Geometry check sheet. Reference: the model listing, model coordinates, mm. A direction names the side the tool comes from. Round coordinates to 2 decimals unless told otherwise and drop trailing zeros. Write each loop counter-clockwise with the first axis right and the second up, starting at its lowest first coordinate (ties: lowest second). Pieces come first, ordered by that corner, then holes. Notation, with made-up numbers: M 40,27 L 56,27 A13 cw 56,50 Z; hole C 56.5,63.5 d8. An arc over 180 degrees is marked long. Answer as CSV lines item,"result". Start each with the question number.
Autodesk Inventor part; units mm, degrees
ref_plane "YZ Plane" through (0, 0, 0) normal (1, 0, 0) x (0, 1, 0)
ref_plane "XZ Plane" through (0, 0, 0) normal (0, 1, 0) x (-1, 0, 0)
ref_plane "XY Plane" through (0, 0, 0) normal (0, 0, 1) x (1, 0, 0)
sketch "Skizze1" plane through (0, 0, 0) normal (0, 0, 1) x (1, 0, 0)
  line L0 (-7, 0) -> (7, 0)
  line L1 (0, -7) -> (0, 7)
  circle A0 centre (0, 0) radius 5
  dimension "d0" = 10
extrude "Extrusion1" add sketch "Skizze1" along normal mid plane 25
sketch "Skizze2" plane through (0, 0, -12.5) normal (0, 0, -1) x (-1, 0, 0)
  circle A0 centre (0, 0) radius 2.5
  dimension "d3" = 5
extrude "Extrusion2" add sketch "Skizze2" along normal blind 15
sketch "Skizze3" plane through (0, 0, 12.5) normal (0, 0, 1) x (1, 0, 0)
  circle A0 centre (0, 0) radius 2.5
  circle A1 centre (0, 0) radius 2.5
extrude "Extrusion3" add sketch "Skizze3" along normal blind 15
thread "Gewinde1"
sketch "Skizze4" plane through (0, 0, 0) normal (1, 0, 0) x (0, 1, 0)
  line L0 (-7, 0) -> (7, 0)
  line L1 (0, -5.6) -> (0, 5.6)
  line L2 (-7, 4) -> (-4, 4)
  line L3 (-4, 4) -> (-4, -4)
  line L4 (-4, -4) -> (-7, -4)
  line L5 (-7, -4) -> (-7, 4)
  line L6 (-7, 4) -> (-4, -4) construction
  line L7 (-4, 4) -> (-7, -4) construction
  line L8 (7, 4) -> (4, 4)
  line L9 (4, 4) -> (4, -4)
  line L10 (4, -4) -> (7, -4)
  line L11 (7, -4) -> (7, 4)
  line L12 (7, 4) -> (4, -4) construction
  line L13 (4, 4) -> (7, -4) construction
  point P0 (0, 0)
  point P1 (-5.5, 0)
  point P2 (5.5, 0)
  dimension "d10" = 8
  dimension "d11" = 8
  dimension "d12" = 3
extrude "Extrusion4" cut sketch "Skizze4" along normal mid plane 20
properties part number "24_0497_0017"
1) Section check D-D, the plane z = -2.5. Record the cut outline in (x, y), plus the area to 3 significant figures.
2) Scan lines: line 1 (Z direction, x = 3, y = -0.5); line 2 (Y direction, x = 0, z = 15); line 3 (X direction, y = 0.25, z = -9.5). Record each from-to range of solid material in increasing order. Write a range as from..to.
3) Mould release check, pull along Z, two halves, no side actions. Record for faces 1 (the cylindrical face through (-5, 0, 0)), 2 (the flat face through (2, -2, -12.5)), 3 (the flat face through (0, -4, 0)): released by +Z, released by -Z, zero draft, split by the parting line, or undercut.
4) Access from +Z, -Z, +X, -X, +Y, -Y to the whole of each face (thin tool, end or side, straight path). Record for faces 4 (the flat face through (0, 4.4, 4)), 5 (the cylindrical face through (0.54, 2.44, -19.9)), 6 (the flat face through (2, -2, 12.5)), 7 (the flat face through (0, -4.4, -4)).
5) Section check A-A, the plane x = 0. Record the cut outline in (y, z).
6) Section check C-C, the plane z = 19.5. Record the cut outline in (x, y), plus the area to 3 significant figures.
7) Go/stop test with flat-tipped pins: pin 1 (1.5 mm diameter, centred on x = -1.5, y = -4, fed in from +Z); pin 2 (3 mm diameter, centred on x = 2.5, z = 21.5, fed in from -Y); pin 3 (4 mm diameter, centred on y = 3.5, z = 10, fed in from +X); pin 4 (2 mm diameter, centred on y = -4, z = -21.5, fed in from -X). Record where each tip stops, or that it passes through.
8) Section check B-B, the plane y = 0. Record the cut outline in (x, z), plus the area to 3 significant figures.
Results:
1,outline,"M -3,-4 L 3,-4 A5 ccw 3,4 L -3,4 A5 ccw Z"
1,area,"70.4 mm^2"
2,line 1,"z = -12.5..12.5"
2,line 2,"y = -2.5..2.5"
2,line 3,"x = -4.99..4.99"
3,face 1,"zero draft"
3,face 2,"released by -Z"
3,face 3,"undercut"
4,face 4,"+X, -X, +Y"
4,face 5,"-Z"
4,face 6,"+Z"
4,face 7,"+X, -X, -Y"
5,outline,"M -5,-12.5 L -2.5,-12.5 L -2.5,-27.5 L 2.5,-27.5 L 2.5,-12.5 L 5,-12.5 L 5,-4 L 4,-4 L 4,4 L 5,4 L 5,12.5 L 2.5,12.5 L 2.5,27.5 L -2.5,27.5 L -2.5,12.5 L -5,12.5 L -5,4 L -4,4 L -4,-4 L -5,-4 Z"
6,outline,"C 0,0 d5"
6,area,"19.6 mm^2"
7,pin 1,"stops at z = 12.5"
7,pin 2,"stops at y = -2.29"
7,pin 3,"stops at x = 4.77"
7,pin 4,"passes through"
8,outline,"M -5,-12.5 L -2.5,-12.5 L -2.5,-27.5 L 2.5,-27.5 L 2.5,-12.5 L 5,-12.5 L 5,12.5 L 2.5,12.5 L 2.5,27.5 L -2.5,27.5 L -2.5,12.5 L -5,12.5 Z"
8,area,"400 mm^2"
